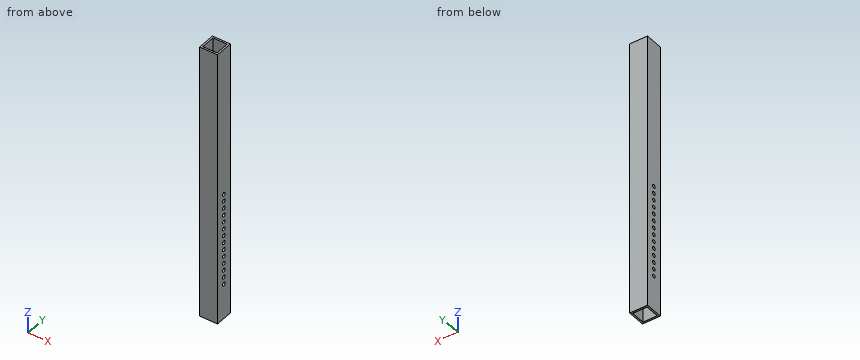
```python
from build123d import *

# Parameters (mm, degrees)
F0_W     = 63.5
F0_H     = 63.5
F0_W_2   = 50.8
F0_H_2   = 50.8
F1_DEPTH = 990.6
F3_D     = 12.7


# Not quite as in the source:
# - a length typed as a fraction of an inch, garbled in the dataset ("3 / 203.2 mm" for 3/8 in), is restored


with BuildPart() as f1:
    # F0 (on Top) → F1 (new body)
    with BuildSketch(Plane.XY):
        Rectangle(F0_W, F0_H)
        Rectangle(F0_W_2, F0_H_2, mode=Mode.SUBTRACT)
    extrude(amount=F1_DEPTH)

    # F3 (through all)
    with Locations(Plane.YZ.offset(31.75)):
        with Locations((0, 127), (0, 152.4), (0, 177.8), (0, 203.2), (0, 228.6), (0, 254), (0, 279.4), (0, 304.8), (0, 330.2), (0, 355.6), (0, 381), (0, 406.4), (0, 431.8), (0, 457.2)):
            Hole(F3_D / 2)


solid = f1.part
```
Read the model definition and answer for the solid it produces. Units are mm, in the model's axes. Give positions to 0.01 mm unless a question says otherwise; leave off trailing zeros. Loops run counter-clockwise (first coordinate to the right, second up) from the corner with the lowest first, then second, coordinate; pieces in that order, holes last.
Item 1: Find the intervals of material crossed by line 1 along Y through (x, z) = (12, 732.5), in increasing order.
Item 2: The part is cut by section B-B (x = 2). Write down the section's boundary in (y, z), and give its area (3 significant figures).
Item 3: The part is cut by section A-A (z = 686). Write down the section's boundary in (x, y), and give its area (3 significant figures).
Taken from the geometry:
1. line 1: y = -31.75 to -25.4, 25.4 to 31.75
2. outline: (-31.75, 0) - (-25.4, 0) - (-25.4, 990.6) - (-31.75, 990.6) - close; (25.4, 0) - (31.75, 0) - (31.75, 990.6) - (25.4, 990.6) - close
2. area: 12,600 mm2
3. outline: (-31.75, -31.75) - (31.75, -31.75) - (31.75, 31.75) - (-31.75, 31.75) - close; hole (-25.4, -25.4) - (25.4, -25.4) - (25.4, 25.4) - (-25.4, 25.4) - close
3. area: 1,450 mm2
